```python
from build123d import *

# Parameters (mm, degrees)
SKETCH3_W           = 610
SKETCH3_H           = 1305
SKETCH3_W_2         = 605.325670498
SKETCH3_H_2         = 1295
BOSS_EXTRUDE2_DEPTH = 640
SKETCH4_R           = 30
SKETCH4_R_2         = 15
CUT_EXTRUDE1_DEPTH  = 640
SKETCH5_W           = 610
SKETCH5_H           = 1305
BOSS_EXTRUDE3_DEPTH = 10


with BuildPart() as part:
    # Sketch3 → Boss-Extrude2 (new body)
    with BuildSketch(Plane(origin=(0, 0, 0), x_dir=(1, 0, 0), z_dir=(0, 1, 0))):
        Rectangle(SKETCH3_W, SKETCH3_H)
        Rectangle(SKETCH3_W_2, SKETCH3_H_2, mode=Mode.SUBTRACT)
    extrude(amount=BOSS_EXTRUDE2_DEPTH)

    # Sketch4 → Cut-Extrude1 (cut)
    with BuildSketch(Plane(origin=(305, 0, 0), x_dir=(0, 0, -1), z_dir=(1, 0, 0))):
        with Locations((-115, 502.5)):
            Circle(SKETCH4_R)
        with Locations((10, 112.5)):
            Circle(SKETCH4_R)
        with Locations((-240, 317.5)):
            Circle(SKETCH4_R_2)
    extrude(amount=-CUT_EXTRUDE1_DEPTH, mode=Mode.SUBTRACT)

    # Sketch5 → Boss-Extrude3 (add)
    with BuildSketch(Plane(origin=(0, 640, 0), x_dir=(1, 0, 0), z_dir=(0, 1, 0))):
        Rectangle(SKETCH5_W, SKETCH5_H)
    extrude(amount=BOSS_EXTRUDE3_DEPTH)


solid = part.part
```
Part model, mm, in its own coordinate system. A direction names the side the tool comes from. Round coordinates to 2 decimals unless told otherwise and drop trailing zeros. Loops run counter-clockwise (first coordinate to the right, second up) from the corner with the lowest first, then second, coordinate; pieces in that order, holes last. Notation, with made-up numbers: (-7.5, 37) -> (6.5, 37) arc R20 cw to (6.5, 54) -> close; hole circle Ø5 at (-7.5, 59.5). An arc over 180 degrees is marked (long way). Use one line per item in the form item = value. Start each with the question number.
Item 1: Drill centre lines: line 1 along Z through (x, y) = (303, 502); line 2 along X through (y, z) = (256, 20.5); line 3 along Y through (x, z) = (-303.85, -10). Where is each one in solid material? Low to high.
Item 2: Two-plate mould, pull along X, no slides. Class faces 3 (the flat face through (-305, 320, 9)), 4 (the cylindrical face through (303.85, 330.15, 231.94)), 5 (the flat face through (302.663, 316, 9)): released by +X, released by -X, zero draft, split by the parting line, or undercut.
Item 3: Band-saw the part on B-B (z = 115). List the corners of the cut face in (x, y).
Item 4: Band-saw the part on C-C (y = 604). List the corners of the cut face in (x, z).
Item 5: Drop a flat-ended pin along its axis: pin 1 Ø1.5 at (x, z) = (53.5, 486.5) entering from -Y. Give the stop position or say it passes through.
Item 6: Band-saw the part on A-A (y = 112.5). List the corners of the cut face in (x, z).
Item 7: Tool access for faces 1 (the cylindrical face through (303.848, 83.213, -3.497)), 2 (the flat face through (-4, 316, 647.5)): list every direction of +Z, -Z, +X, -X, +Y, -Y with a clear straight run to the whole face (end or side of a thin tool).
Item 8: Band-saw the part on D-D (z = -181). List the corners of the cut face in (x, y).
Data:
q1.line_1 = -652.5 to 85, 145 to 652.5
q1.line_2 = -305 to -302.66, 302.66 to 305
q1.line_3 = 0 to 82.5, 142.5 to 650
q2.face_3 = released by -X
q2.face_4 = zero draft
q2.face_5 = undercut
q3.outline = (-305, 0) -> (-302.66, 0) -> (-302.66, 472.5) -> (-305, 472.5) -> close; (-305, 532.5) -> (-302.66, 532.5) -> (-302.66, 640) -> (302.66, 640) -> (302.66, 532.5) -> (305, 532.5) -> (305, 650) -> (-305, 650) -> close; (302.66, 0) -> (305, 0) -> (305, 472.5) -> (302.66, 472.5) -> close
q4.outline = (-305, -652.5) -> (305, -652.5) -> (305, 652.5) -> (-305, 652.5) -> close; hole (-302.66, -647.5) -> (302.66, -647.5) -> (302.66, 647.5) -> (-302.66, 647.5) -> close
q5.pin_1 = 640
q6.outline = (-305, -652.5) -> (305, -652.5) -> (305, -40) -> (302.66, -40) -> (302.66, -647.5) -> (-302.66, -647.5) -> (-302.66, -40) -> (-305, -40) -> close; (-305, 20) -> (-302.66, 20) -> (-302.66, 647.5) -> (302.66, 647.5) -> (302.66, 20) -> (305, 20) -> (305, 652.5) -> (-305, 652.5) -> close
q7.face_1 = +X, -X
q7.face_2 = -Y
q8.outline = (-305, 0) -> (-302.66, 0) -> (-302.66, 640) -> (302.66, 640) -> (302.66, 0) -> (305, 0) -> (305, 650) -> (-305, 650) -> close
